Here's how the part is built. I have some questions about the finished solid (model axes, mm). A direction names the side the tool comes from. Give positions to 0.01 mm unless a question says otherwise; leave off trailing zeros. Write each loop counter-clockwise with the first axis right and the second up, starting at its lowest first coordinate (ties: lowest second). Pieces come first, ordered by that corner, then holes. Notation, with made-up numbers: (-33, 62) -> (23, 62) arc R8 cw to (23, 66) -> close; hole circle Ø11 at (-9, -39.75). An arc over 180 degrees is marked (long way). Put each result on its own line as item: value. Start each with the question number.
from build123d import *

# Parameters (mm, degrees)
F0_W     = 50.8
F0_H     = 50.8
F0_R     = 12.7
F1_DEPTH = 50.8
F2_W     = 50.8
F2_H     = 50.8
F2_R     = 12.7
F3_DEPTH = 25.4


with BuildPart() as f1:
    # F0 (on Front) → F1 (new body)
    with BuildSketch(Plane.XZ):
        with Locations((25.4, 25.4)):
            Rectangle(F0_W, F0_H)
        with Locations((25.4, 25.4)):
            Circle(F0_R, mode=Mode.SUBTRACT)
    extrude(amount=F1_DEPTH)

    # F2 (on face) → F3 (join)
    with BuildSketch(Plane.YZ.offset(50.8)):
        with Locations((-25.4, 25.4)):
            Rectangle(F2_W, F2_H)
        with Locations((-25.4, 25.4)):
            Circle(F2_R, mode=Mode.SUBTRACT)
    extrude(amount=F3_DEPTH)


solid = f1.part
1) I want a section at D-D, the plane x = 53. Write out the boundary of the cut face in (y, z).
2) I need wall thicknesses on probe 1 along Y at (x, z) = (70, 25); probe 2 along Z at (x, y) = (25, -28); probe 3 along X at (y, z) = (-17, 29.5). Which ranges of each line are inside material? Lowest first, please.
3) Which directions (+Z, -Z, +X, -X, +Y, -Y) give clear straight access to the entire face, cutting with the end or side of a thin tool? Please do faces 5 (the flat face through (0, -25, 25)), 6 (the flat face through (50.8, -25, 25)).
4) Thinking about a two-plate mould opening in Y: for faces 1 (the flat face through (38, -50.8, 31)), 2 (the cylindrical face through (63.322, -18.573, 36.109)), 3 (the flat face through (38, 0, 31)), 4 (the flat face through (38, -26, 0)), which applies, released by +Y, released by -Y, zero draft, split by the parting line, or undercut?
5) I want a section at B-B, the plane x = 25.4. Write out the boundary of the cut face in (y, z), and give its area (3 significant figures).
6) I'm going to push a flat-ended pin straight in: pin 1 Ø7.5 at (y, z) = (-29, 30) entering from +X. Where does the tip first touch, or does it pass through?
7) I want a section at C-C, the plane y = -25.4. Write out the boundary of the cut face in (x, z), and give its area (3 significant figures).
8) I want a section at A-A, the plane z = 25.4. Write out the boundary of the cut face in (x, y), and give its area (3 significant figures).
Established:
1. outline: (-50.8, 0) -> (0, 0) -> (0, 50.8) -> (-50.8, 50.8) -> close; hole circle Ø25.4 at (-25.4, 25.4)
2. probe 1: y = -50.8 to -38.09, -12.71 to 0
2. probe 2: z = 0 to 12.71, 38.09 to 50.8
2. probe 3: x = 0 to 13.38, 37.42 to 50.8
3. face 5: +Z, -Z, -X, +Y, -Y
3. face 6: +X
4. face 1: released by -Y
4. face 2: undercut
4. face 3: released by +Y
4. face 4: zero draft
5. outline: (-50.8, 0) -> (0, 0) -> (0, 12.7) -> (-50.8, 12.7) -> close; (-50.8, 38.1) -> (0, 38.1) -> (0, 50.8) -> (-50.8, 50.8) -> close
5. area: 1,290 mm2
6. pin 1: stops at x = 50.8
7. outline: (0, 0) -> (76.2, 0) -> (76.2, 12.7) -> (50.8, 12.7) -> (50.8, 38.1) -> (76.2, 38.1) -> (76.2, 50.8) -> (0, 50.8) -> close; hole circle Ø25.4 at (25.4, 25.4)
7. area: 2,720 mm2
8. outline: (0, -50.8) -> (12.7, -50.8) -> (12.7, 0) -> (0, 0) -> close; (38.1, -50.8) -> (76.2, -50.8) -> (76.2, -38.1) -> (50.8, -38.1) -> (50.8, -12.7) -> (76.2, -12.7) -> (76.2, 0) -> (38.1, 0) -> close
8. area: 1,940 mm2
